```python
from build123d import *

# Parameters (mm, degrees)
SKETCH1_W               = 152.4
SKETCH1_H               = 127
BOSS_EXTRUDE1_DEPTH     = 2.3622
FILLET1_R               = 2.54
SKETCH9_R               = 4.15
CUT_EXTRUDE8_DEPTH      = 100.218294628
CUT_EXTRUDE11_DEPTH     = 100.218294628
CUT_EXTRUDE12_DEPTH     = 100.218294628
SKETCH16_R              = 4.15
CUT_EXTRUDE14_DEPTH     = 100.218294628
SKETCH17_R              = 2.7305
CUT_EXTRUDE16_DEPTH     = 100.218294628
MIRROR7_COPY_1_SKETCH_R = 2.7305
MIRROR7_COPY_1_DEPTH    = 100.218294628
SKETCH26_W              = 10.16
SKETCH26_H              = 12.7
CUT_EXTRUDE26_DEPTH     = 100.218294628
SKETCH27_R              = 4.15
CUT_EXTRUDE27_DEPTH     = 100.218294628
SKETCH29_R              = 4.15
CUT_EXTRUDE28_DEPTH     = 100.218294628
SKETCH30_R              = 4.15
CUT_EXTRUDE29_DEPTH     = 100.218294628
SKETCH31_R              = 4.15
CUT_EXTRUDE30_DEPTH     = 100.218294628


with BuildPart() as part:
    # Sketch1 → Boss-Extrude1 (new body)
    with BuildSketch(Plane(origin=(0, 0, 0), x_dir=(1, 0, 0), z_dir=(0, 1, 0))):
        Rectangle(SKETCH1_W, SKETCH1_H)
    extrude(amount=BOSS_EXTRUDE1_DEPTH)

    # Fillet1
    fillet1_edges = [part.edges().sort_by_distance(p)[0] for p in [
        (76.2, 1.1811, 63.5),
        (-76.2, 1.1811, 63.5),
        (-76.2, 1.1811, -63.5),
        (76.2, 1.1811, -63.5),
    ]]
    fillet(fillet1_edges, radius=FILLET1_R)

    # Sketch9 → Cut-Extrude8 (cut, through all)
    with BuildSketch(Plane.XZ):
        with Locations(Location((60.8584, 27.94, 0), (0, 0, 270))):
            Circle(SKETCH9_R)
        with Locations(Location((60.8584, -2.54, 0), (0, 0, 270))):
            Circle(SKETCH9_R)
    extrude(amount=-CUT_EXTRUDE8_DEPTH, mode=Mode.SUBTRACT)

    # Sketch12 → Cut-Extrude11 (cut, through all)
    with BuildSketch(Plane.XZ):
        with BuildLine():
            Line((-3.81, 59.465627528), (3.81, 59.465627528))
            ThreePointArc((3.81, 59.465627528), (8.387405636, 54.888221892), (3.81, 50.310816255))
            Line((3.81, 50.310816255), (-3.81, 50.310816255))
            ThreePointArc((-3.81, 50.310816255), (-8.387405636, 54.888221892), (-3.81, 59.465627528))
        make_face()
    cut_extrude11 = extrude(amount=-CUT_EXTRUDE11_DEPTH, mode=Mode.SUBTRACT)

    # Mirror3: Cut-Extrude11 across plane
    add(cut_extrude11.mirror(Plane.XY), mode=Mode.SUBTRACT)

    # Sketch13 → Cut-Extrude12 (cut, through all)
    with BuildSketch(Plane(origin=(0, 0, 0), x_dir=(-1, 0, 0), z_dir=(0, -1, 0))):
        with BuildLine():
            Line((60.052874771, -45.72), (60.052874771, -53.34))
            ThreePointArc((60.052874771, -53.34), (55.88, -57.512874771), (51.707125229, -53.34))
            Line((51.707125229, -53.34), (51.707125229, -45.72))
            ThreePointArc((51.707125229, -45.72), (55.88, -41.547125229), (60.052874771, -45.72))
        make_face()
    extrude(amount=-CUT_EXTRUDE12_DEPTH, mode=Mode.SUBTRACT)

    # Sketch16 → Cut-Extrude14 (cut, through all)
    with BuildSketch(Plane(origin=(0, 0, 0), x_dir=(-1, 0, 0), z_dir=(0, -1, 0))):
        with Locations(Location((-69.599893995, 19.704320306, 0), (0, 0, 90))):
            Circle(SKETCH16_R)
        with Locations(Location((-46.522565834, 32.264238523, 0), (0, 0, 90))):
            Circle(SKETCH16_R)
    extrude(amount=-CUT_EXTRUDE14_DEPTH, mode=Mode.SUBTRACT)

    # Sketch17 → Cut-Extrude16 (cut, through all)
    with BuildSketch(Plane.XZ):
        with Locations(Location((71.794813785, 59.510435834, 0), (0, 0, 270))):
            Circle(SKETCH17_R)
    cut_extrude16 = extrude(amount=-CUT_EXTRUDE16_DEPTH, mode=Mode.SUBTRACT)

    # Mirror6: Cut-Extrude16 across plane
    add(cut_extrude16.mirror(Plane(origin=(0, 0, 0), x_dir=(0, 0, 1), z_dir=(1, 0, 0))), mode=Mode.SUBTRACT)

    # Mirror7: Cut-Extrude16 across plane
    add(cut_extrude16.mirror(Plane.XY), mode=Mode.SUBTRACT)

    # Mirror7 copy 1 sketch → Mirror7 copy 1 (cut, through all)
    with BuildSketch(Plane(origin=(0, 0, 0), x_dir=(-1, 0, 0), z_dir=(0, -1, 0))):
        with Locations(Location((71.794813785, 59.510435834, 0), (0, 0, 270))):
            Circle(MIRROR7_COPY_1_SKETCH_R)
    extrude(amount=-MIRROR7_COPY_1_DEPTH, mode=Mode.SUBTRACT)

    # Sketch26 → Cut-Extrude26 (cut, through all)
    with BuildSketch(Plane(origin=(0, 2.3622, 0), x_dir=(1, 0, 0), z_dir=(0, 1, 0))):
        with Locations((35.56, 0)):
            Rectangle(SKETCH26_W, SKETCH26_H)
    extrude(amount=-CUT_EXTRUDE26_DEPTH, mode=Mode.SUBTRACT)

    # Sketch27 → Cut-Extrude27 (cut, through all)
    with BuildSketch(Plane.XZ):
        with Locations(Location((-60.09170874, 33.02, 0), (0, 0, 270))):
            Circle(SKETCH27_R)
        with Locations(Location((-50.09170874, -30.48, 0), (0, 0, 270))):
            Circle(SKETCH27_R)
    extrude(amount=-CUT_EXTRUDE27_DEPTH, mode=Mode.SUBTRACT)

    # Sketch29 → Cut-Extrude28 (cut, through all)
    with BuildSketch(Plane(origin=(0, 2.3622, 0), x_dir=(1, 0, 0), z_dir=(0, 1, 0))):
        with Locations(Location((35.56, 19.681240592, 0), (0, 0, 270))):
            Circle(SKETCH29_R)
        with Locations(Location((35.56, -19.681240592, 0), (0, 0, 270))):
            Circle(SKETCH29_R)
    extrude(amount=-CUT_EXTRUDE28_DEPTH, mode=Mode.SUBTRACT)

    # Sketch30 → Cut-Extrude29 (cut, through all)
    with BuildSketch(Plane(origin=(0, 2.3622, 0), x_dir=(1, 0, 0), z_dir=(0, 1, 0))):
        with Locations(Location((69.803274088, -46.355, 0), (0, 0, 270))):
            Circle(SKETCH30_R)
        with Locations(Location((30.63517528, -46.355, 0), (0, 0, 270))):
            Circle(SKETCH30_R)
    cut_extrude29 = extrude(amount=-CUT_EXTRUDE29_DEPTH, mode=Mode.SUBTRACT)

    # Mirror8: Cut-Extrude29 across plane
    add(cut_extrude29.mirror(Plane.XY), mode=Mode.SUBTRACT)

    # Sketch31 → Cut-Extrude30 (cut, through all)
    with BuildSketch(Plane(origin=(0, 2.3622, 0), x_dir=(1, 0, 0), z_dir=(0, 1, 0))):
        with Locations(Location((-62.942335235, -12.79551579, 0), (0, 0, 270))):
            Circle(SKETCH31_R)
        with Locations(Location((-62.942335235, 13.549600091, 0), (0, 0, 270))):
            Circle(SKETCH31_R)
    extrude(amount=-CUT_EXTRUDE30_DEPTH, mode=Mode.SUBTRACT)


solid = part.part
```
Geometry: final body of the model. Coordinates: model frame, mm. Round coordinates to 2 decimals unless told otherwise and drop trailing zeros. Write each loop counter-clockwise with the first axis right and the second up, starting at its lowest first coordinate (ties: lowest second). Pieces come first, ordered by that corner, then holes. Notation, with made-up numbers: M 77,42 L 111,42 A30 cw 111,68 Z; hole C 22.5,39.25 d9. An arc over 180 degrees is marked long. Answer in a Markdown table with one row per item. Add a question column.
(1) Cut plane D-D, the plane z = -12. Return the cut outline in (x, y), then the cut area to 3 significant figures.
(2) Contact query for a flat-ended pin moving along its axis: pin 1 (5 mm diameter, centred on x = 69.8, z = 46.36, fed in from +Y). Output: stop coordinate, or through.
(3) Ray query, L1, parallel to Z at x = -2.5, y = 0.1; L2, parallel to X at y = 1.8, z = -1; L3, parallel to Z at x = -4.5, y = 1.55. Return the intervals inside material, ascending.
(4) Cut plane C-C, the plane y = 1.8. Give the number of separate pieces and of enclosed holes in the cut face, then the cut area to 3 significant figures.
(5) Cut plane B-B, the plane z = -30.48. Return the cut outline in (x, y), then the cut area to 3 significant figures.
(6) Draft query along Z for faces 1 (the face through (-8.386, 1.165, 54.788)), 2 (the face through (-1, 0, -1)). Return one class per face: pulls with the +Z half, pulls with the -Z half, needs draft (parallel to the pull), parting line crosses it, or undercut.
(7) Cut plane A-A, the plane z = 27. Return the cut outline in (x, y).
Established:
| question | item | result |
|---|---|---|
| 1 | outline | M -76.2,0 L -66.79,0 L -66.79,2.36 L -76.2,2.36 Z; M -59.09,0 L 76.2,0 L 76.2,2.36 L -59.09,2.36 Z |
| 1 | area | 342 mm² |
| 2 | pin 1 | through |
| 3 | L1 | -63.5 to -59.47, -50.31 to 50.31, 59.47 to 63.5 |
| 3 | L2 | -76.2 to 30.48, 40.64 to 57, 64.71 to 76.2 |
| 3 | L3 | -63.5 to -59.41, -50.36 to 50.36, 59.41 to 63.5 |
| 4 | separate pieces | 1 |
| 4 | enclosed holes | 22 |
| 4 | area | 18,000 mm² |
| 5 | outline | M -76.2,0 L -54.24,0 L -54.24,2.36 L -76.2,2.36 Z; M -45.94,0 L 42.78,0 L 42.78,2.36 L -45.94,2.36 Z; M 50.27,0 L 76.2,0 L 76.2,2.36 L 50.27,2.36 Z |
| 5 | area | 323 mm² |
| 6 | face 1 | undercut |
| 6 | face 2 | needs draft |
| 7 | outline | M -76.2,0 L 56.82,0 L 56.82,2.36 L -76.2,2.36 Z; M 64.9,0 L 76.2,0 L 76.2,2.36 L 64.9,2.36 Z |
